Part model, mm, in its own coordinate system. Face numbers are marked on the shaded views. A direction names the side the tool comes from. Give positions to 0.01 mm unless a question says otherwise; leave off trailing zeros. Order: outer loops, then holes, each group sorted by start corner. A loop starts at its lowest first (then second) coordinate and runs counter-clockwise, first axis right, second up. Notation, with made-up numbers: M 1,-33.75 L 13,-33.75 A10 ccw 13,-17.75 Z; hole C -4.75,70.5 d2. An arc over 180 degrees is marked long. Return JSON: item names as keys, results as strings.
from build123d import *

# Parameters (mm, degrees)
SKETCH1_W               = 80
SKETCH1_H               = 119
BOSS_EXTRUDE1_DEPTH     = 32
SKETCH2_W               = 78
SKETCH2_H               = 115
CUT_EXTRUDE1_DEPTH      = 30
CUT_EXTRUDE2_DEPTH      = 130.55693729
CUT_EXTRUDE2_DEPTH_BACK = 130.55693729
SKETCH3_R               = 2.5
SKETCH4_W               = 47.7
SKETCH4_H               = 28.2
CUT_EXTRUDE4_DEPTH      = 10
CUT_EXTRUDE5_START      = -1
SKETCH5_W               = 5
SKETCH5_H               = 48.939685833
CUT_EXTRUDE5_DEPTH      = 30
SKETCH6_W               = 4
SKETCH6_H               = 16.969842916
SKETCH6_H_2             = 16.969842917
CUT_EXTRUDE6_DEPTH      = 2
SKETCH7_R               = 2.3
CUT_EXTRUDE7_DEPTH      = 79.51273782


with BuildPart() as part:
    # Sketch1 → Boss-Extrude1 (new body)
    with BuildSketch(Plane(origin=(0, 0, 0), x_dir=(1, 0, 0), z_dir=(0, 1, 0))):
        Rectangle(SKETCH1_W, SKETCH1_H)
    extrude(amount=BOSS_EXTRUDE1_DEPTH)

    # Sketch2 → Cut-Extrude1 (cut)
    with BuildSketch(Plane(origin=(0, 32, 0), x_dir=(1, 0, 0), z_dir=(0, 1, 0))):
        with Locations((1, 0)):
            Rectangle(SKETCH2_W, SKETCH2_H)
    extrude(amount=-CUT_EXTRUDE1_DEPTH, mode=Mode.SUBTRACT)

    # Sketch3 → Cut-Extrude2 (cut, two sides: drawn at the far end of the back side and taken through both)
    with BuildSketch(Plane.XY.offset(59.5).offset(-CUT_EXTRUDE2_DEPTH_BACK)):
        with Locations((30, 14.5)):
            Circle(SKETCH3_R)
    extrude(amount=CUT_EXTRUDE2_DEPTH + CUT_EXTRUDE2_DEPTH_BACK, mode=Mode.SUBTRACT)

    # Sketch4 → Cut-Extrude4 (cut)
    with BuildSketch(Plane(origin=(-38, 0, 0), x_dir=(0, 0, -1), z_dir=(1, 0, 0))):
        with Locations((-31.205661858, 16)):
            Rectangle(SKETCH4_W, SKETCH4_H)
    extrude(amount=-CUT_EXTRUDE4_DEPTH, mode=Mode.SUBTRACT)

    # Sketch5 → Cut-Extrude5 (cut)
    with BuildSketch(Plane(origin=(0, 2, 0), x_dir=(1, 0, 0), z_dir=(0, 1, 0)).offset(CUT_EXTRUDE5_START)):
        with Locations((-36.5, -30.585818942)):
            Rectangle(SKETCH5_W, SKETCH5_H)
    extrude(amount=CUT_EXTRUDE5_DEPTH, mode=Mode.SUBTRACT)

    # Sketch6 → Cut-Extrude6 (cut)
    with BuildSketch(Plane(origin=(0, 1, 0), x_dir=(1, 0, 0), z_dir=(0, 1, 0))):
        with Locations((-36, -14.600897483)):
            Rectangle(SKETCH6_W, SKETCH6_H)
        with Locations((-36, -46.570740399)):
            Rectangle(SKETCH6_W, SKETCH6_H_2)
    extrude(amount=-CUT_EXTRUDE6_DEPTH, mode=Mode.SUBTRACT)

    # Sketch7 → Cut-Extrude7 (cut, through all)
    with BuildSketch(Plane.XZ):
        with Locations(Location((30, 25, 0), (0, 0, 270))):
            Circle(SKETCH7_R)
        with Locations(Location((30, -25, 0), (0, 0, 270))):
            Circle(SKETCH7_R)
    extrude(amount=-CUT_EXTRUDE7_DEPTH, mode=Mode.SUBTRACT)


solid = part.part
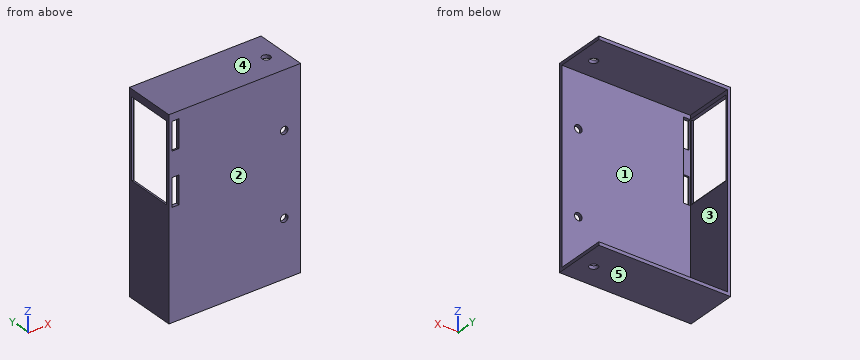
Q1. Two-plate mould, pull along Z, no slides. Class the marked faces 3, 4 and 5: +Z half, -Z half, draft (parallel to the pull), parting line (faces both ways), or undercut.
Established:
{"face 3": "undercut", "face 4": "+Z half", "face 5": "-Z half"}
Q2. Band-saw the part on D-D (z = 25). Give the cut face in (x, y).
Established:
{"outline": "M -40,0 L 27.7,0 L 27.7,2 L -34,2 L -34,1 L -39,1 L -39,1.9 L -40,1.9 Z; M -40,30.1 L -39,30.1 L -39,31 L -38,31 L -38,32 L -40,32 Z; M 32.3,0 L 40,0 L 40,2 L 32.3,2 Z"}
Q3. Band-saw the part on C-C (y = 14.5). Give the cut face in (x, z), then the cut area to 3 significant figures.
Established:
{"outline": "M -40,-59.5 L 27.5,-59.5 L 27.5,-57.5 L -38,-57.5 L -38,6.12 L -39,6.12 L -39,7.36 L -40,7.36 Z; M -40,55.06 L -38,55.06 L -38,57.5 L 27.5,57.5 L 27.5,59.5 L -40,59.5 Z; M 32.5,-59.5 L 40,-59.5 L 40,-57.5 L 32.5,-57.5 Z; M 32.5,57.5 L 40,57.5 L 40,59.5 L 32.5,59.5 Z", "area": "433 mm²"}
Q4. Probe line 1 along Z through (x, y) = (36.5, 27.5); line 2 along X through (y, z) = (1, -25); line 3 along Y through (x, z) = (30, 58). List the from-to ranges inside material, lowest first.
Established:
{"line 1": "z = -59.5 to -57.5, 57.5 to 59.5", "line 2": "x = -40 to 27.7, 32.3 to 40", "line 3": "y = 0 to 12, 17 to 32"}
Q5. Band-saw the part on B-B (x = 30). Give the cut face in (y, z).
Established:
{"outline": "M 0,-59.5 L 12,-59.5 L 12,-57.5 L 2,-57.5 L 2,-27.3 L 0,-27.3 Z; M 0,-22.7 L 2,-22.7 L 2,22.7 L 0,22.7 Z; M 0,27.3 L 2,27.3 L 2,57.5 L 12,57.5 L 12,59.5 L 0,59.5 Z; M 17,-59.5 L 32,-59.5 L 32,-57.5 L 17,-57.5 Z; M 17,57.5 L 32,57.5 L 32,59.5 L 17,59.5 Z"}
Q6. Pin check, flat tips, straight feed: pin 1 (8 mm diameter, centred on x = -18, z = -6, fed in from +Y); pin 2 (15 mm diameter, centred on y = 16, z = 7, fed in from +X). Stop position of each tip, or through.
Established:
{"pin 1": "stops at y = 2", "pin 2": "stops at x = -38"}
Q7. Band-saw the part on A-A (z = -25). Give the cut face in (x, y), then the cut area to 3 significant figures.
Established:
{"outline": "M -40,0 L 27.7,0 L 27.7,2 L -38,2 L -38,32 L -40,32 Z; M 32.3,0 L 40,0 L 40,2 L 32.3,2 Z", "area": "211 mm²"}
Q8. 3-axis set-ups, long thin cutter, end or side, ignore diameter. For the marked faces 1 and 2: which of +Z, -Z, +X, -X, +Y, -Y reach the whole face in a straight line?
Established:
{"face 1": "+X, +Y", "face 2": "+Z, -Z, +X, -X, -Y"}
